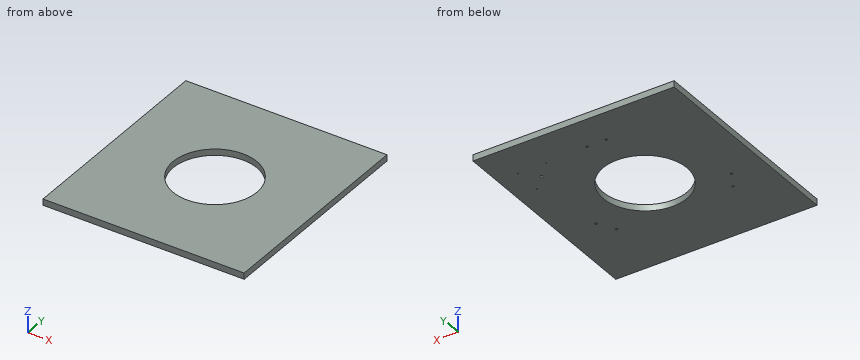
```python
from build123d import *

# Parameters (mm, degrees)
SKETCH1_W           = 480
SKETCH1_H           = 511
BOSS_EXTRUDE1_DEPTH = 15
SKETCH3_R           = 100
CUT_EXTRUDE2_DEPTH  = 15
SKETCH4_R           = 1.5
CUT_EXTRUDE3_DEPTH  = 7
CUT_EXTRUDE4_DEPTH  = 2.3
SKETCH6_R           = 3
CUT_EXTRUDE5_DEPTH  = 7
SKETCH7_R           = 1.5
CUT_EXTRUDE6_DEPTH  = 5


with BuildPart() as part:
    # Sketch1 → Boss-Extrude1 (new body)
    with BuildSketch(Plane.XY):
        Rectangle(SKETCH1_W, SKETCH1_H)
    extrude(amount=BOSS_EXTRUDE1_DEPTH)

    # Sketch3 → Cut-Extrude2 (cut)
    with BuildSketch(Plane(origin=(0, 0, 0), x_dir=(-1, 0, 0), z_dir=(0, 0, -1))):
        Circle(SKETCH3_R)
    extrude(amount=-CUT_EXTRUDE2_DEPTH, mode=Mode.SUBTRACT)

    # Sketch4 → Cut-Extrude3 (cut)
    with BuildSketch(Plane(origin=(0, 0, 0), x_dir=(-1, 0, 0), z_dir=(0, 0, -1))):
        with Locations((22.80945209, 173.254989525)):
            Circle(SKETCH4_R)
        with Locations(Location((-22.80945209, 173.254989525, 0), (0, 0, 180))):
            Circle(SKETCH4_R)
        with Locations((-161.447948306, -66.873929806)):
            Circle(SKETCH4_R)
        with Locations(Location((-138.638496216, -106.381059719, 0), (0, 0, 180))):
            Circle(SKETCH4_R)
        with Locations((138.638496216, -106.381059719)):
            Circle(SKETCH4_R)
        with Locations(Location((161.447948306, -66.873929806, 0), (0, 0, 180))):
            Circle(SKETCH4_R)
    extrude(amount=-CUT_EXTRUDE3_DEPTH, mode=Mode.SUBTRACT)

    # Sketch5 → Cut-Extrude4 (cut)
    with BuildSketch(Plane(origin=(0, 0, 0), x_dir=(-1, 0, 0), z_dir=(0, 0, -1))):
        Polygon((22.80945209, 176.430416006), (20.05945209, 174.842702765), (20.05945209, 171.667276285), (22.80945209, 170.079563045), (25.55945209, 171.667276285), (25.55945209, 174.842702765), align=None)
        Polygon((-20.05945209, 174.842702765), (-20.05945209, 171.667276285), (-22.80945209, 170.079563045), (-25.55945209, 171.667276285), (-25.55945209, 174.842702765), (-22.80945209, 176.430416006), align=None)
        Polygon((-164.197948306, -68.461643046), (-161.447948306, -70.049356286), (-158.697948306, -68.461643046), (-158.697948306, -65.286216566), (-161.447948306, -63.698503325), (-164.197948306, -65.286216566), align=None)
        Polygon((-138.638496216, -109.5564862), (-141.388496216, -107.96877296), (-141.388496216, -104.793346479), (-138.638496216, -103.205633239), (-135.888496216, -104.793346479), (-135.888496216, -107.96877296), align=None)
        Polygon((141.388496216, -107.96877296), (141.388496216, -104.793346479), (138.638496216, -103.205633239), (135.888496216, -104.793346479), (135.888496216, -107.96877296), (138.638496216, -109.5564862), align=None)
        Polygon((164.197948306, -65.286216566), (164.197948306, -68.461643046), (161.447948306, -70.049356286), (158.697948306, -68.461643046), (158.697948306, -65.286216566), (161.447948306, -63.698503325), align=None)
    extrude(amount=-CUT_EXTRUDE4_DEPTH, mode=Mode.SUBTRACT)

    # Sketch6 → Cut-Extrude5 (cut)
    with BuildSketch(Plane(origin=(0, 0, 0), x_dir=(-1, 0, 0), z_dir=(0, 0, -1))):
        with Locations((-156.911542489, 135.010250847)):
            Circle(SKETCH6_R)
    extrude(amount=-CUT_EXTRUDE5_DEPTH, mode=Mode.SUBTRACT)

    # Sketch7 → Cut-Extrude6 (cut)
    with BuildSketch(Plane(origin=(0, 0, 0), x_dir=(-1, 0, 0), z_dir=(0, 0, -1))):
        with Locations((-123.323970382, 168.597822953)):
            Circle(SKETCH7_R)
        with Locations((-190.499114595, 168.597822953)):
            Circle(SKETCH7_R)
        with Locations((-190.499114595, 101.422678741)):
            Circle(SKETCH7_R)
    extrude(amount=-CUT_EXTRUDE6_DEPTH, mode=Mode.SUBTRACT)


solid = part.part
```
The listing builds one solid part. Answer for the finished solid, in the listing's coordinates (mm). Give positions to 0.01 mm unless a question says otherwise; leave off trailing zeros. Write each loop counter-clockwise with the first axis right and the second up, starting at its lowest first coordinate (ties: lowest second). Pieces come first, ordered by that corner, then holes. Notation, with made-up numbers: (-20.5, 65) -> (33.5, 65) arc R23 ccw to (33.5, 86) -> close; hole circle Ø1 at (15, 33.5). An arc over 180 degrees is marked (long way). Use one line per item in the form item = value.
1) Section A-A on x = 0 is taken. Write down the section's boundary in (y, z).
Result:
outline = (-255.5, 0) -> (-100, 0) -> (-100, 15) -> (-255.5, 15) -> close; (100, 0) -> (255.5, 0) -> (255.5, 15) -> (100, 15) -> close
2) Straight lines are drawn through the part: probe 1 along Y at (x, z) = (5.5, 4.5); probe 2 along Y at (x, z) = (44.5, 13.25). For each, find the intervals that lie inside material, in ascending order.
Result:
probe_1 = -255.5 to -99.85, 99.85 to 255.5
probe_2 = -255.5 to -89.55, 89.55 to 255.5
3) Section B-B on y = 0 is taken. Write down the section's boundary in (x, z), plus the area to 3 significant figures.
Result:
outline = (-240, 0) -> (-100, 0) -> (-100, 15) -> (-240, 15) -> close; (100, 0) -> (240, 0) -> (240, 15) -> (100, 15) -> close
area = 4,200 mm²
4) Section C-C on z = 11.5 is taken. Write down the section's boundary in (x, y), plus the area to 3 significant figures.
Result:
outline = (-240, -255.5) -> (240, -255.5) -> (240, 255.5) -> (-240, 255.5) -> close; hole circle Ø200 at (0, 0)
area = 214,000 mm²
5) This flat-tipped pin is pushed along its axis until it touches: P1, Ø1.5, axis at x = 138, y = -106.5, coming from the -Z side. Where does it stop, or does it pass through?
Result:
P1 = 7
